For this review, take the finished solid that the model builds, in its own axes (mm). Face numbers are marked on the shaded views. Coordinates: 2 decimals unless noted, no trailing zeros. Write each loop counter-clockwise with the first axis right and the second up, starting at its lowest first coordinate (ties: lowest second). Pieces come first, ordered by that corner, then holes.
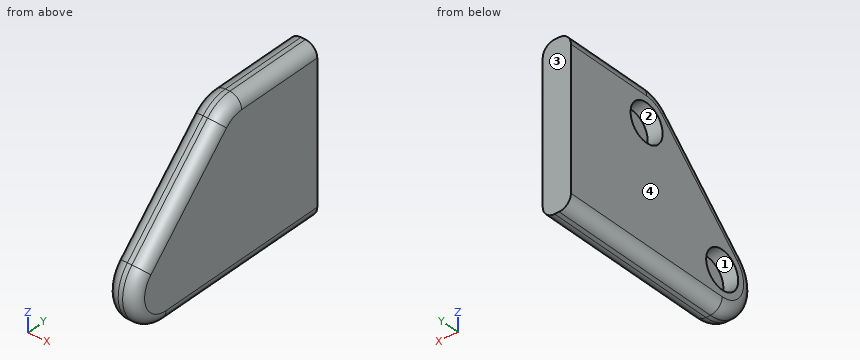
```python
from build123d import *

# Parameters (mm, degrees)
F1_DEPTH = 19
F2_R     = 12.7
F3_DEPTH = 10
F4_R     = 8
F5_R     = 8


with BuildPart() as f1:
    # F0 (on Right) → F1 (new body)
    with BuildSketch(Plane.YZ):
        with BuildLine():
            Line((-120, 0), (0, 0))
            Line((0, 0), (0, 110))
            Line((0, 110), (-60, 110))
            ThreePointArc((-60, 110), (-69.567086, 108.096988), (-77.67767, 102.67767))
            Line((-77.67767, 102.67767), (-137.67767, 42.67767))
            ThreePointArc((-137.67767, 42.67767), (-143.096988, 15.432914), (-120, 0))
        make_face()
    extrude(amount=F1_DEPTH)

    # F2 (on face) → F3 (cut)
    with BuildSketch(Plane(origin=(0, 0, 0), x_dir=(0, -1, 0), z_dir=(-1, 0, 0))):
        with Locations((60, 85)):
            Circle(F2_R)
        with Locations((120, 25)):
            Circle(F2_R)
    extrude(amount=-F3_DEPTH, mode=Mode.SUBTRACT)

    # F4
    f4_edges = [f1.edges().sort_by_distance(p)[0] for p in [
        (0, -30, 110),
    ]]
    fillet(f4_edges, radius=F4_R)

    # F5
    f5_edges = [f1.edges().sort_by_distance(p)[0] for p in [
        (19, -30, 110),
    ]]
    fillet(f5_edges, radius=F5_R)


solid = f1.part
```
Q1. Add section A-A (x = 1.5). State the section outline as (y, z) points, then the cut area to 3 significant figures.
Ans:
outline: (-135.32, 40.32) arc R21.66 ccw to (-120, 3.34) - (0, 3.34) - (0, 106.66) - (-60, 106.66) arc R21.66 ccw to (-75.32, 100.32) - close; hole circle Ø25.4 at (-120, 25); hole circle Ø25.4 at (-60, 85)
area: 10,900 mm2
Q2. Draft analysis for pull direction Y (two halves, no side actions). For the marked faces 1, 2, 3 and 4, state which applies: +Y half, -Y half, draft (parallel to the pull), parting line (faces both ways), or undercut.
Ans:
face 1: undercut
face 2: undercut
face 3: +Y half
face 4: draft
Q3. Add section B-B (y = -40.5). State the section outline as (x, z) points, then the cut area to 3 significant figures.
Ans:
outline: (0, 8) arc R8 ccw to (8, 0) - (11, 0) arc R8 ccw to (19, 8) - (19, 102) arc R8 ccw to (11, 110) - (8, 110) arc R8 ccw to (0, 102) - close
area: 2,040 mm2
Q4. Add section C-C (x = 17.5). State the section outline as (y, z) points.
Ans:
outline: (-135.32, 40.32) arc R21.66 ccw to (-120, 3.34) - (0, 3.34) - (0, 106.66) - (-60, 106.66) arc R21.66 ccw to (-75.32, 100.32) - close
Q5. Clearance check with flat-ended pins moving along their axes: pin 1 Ø6 at (y, z) = (-63, 84.5) entering from -X; pin 2 Ø12 at (y, z) = (-70, 91) entering from -X; pin 3 Ø3 at (x, z) = (6, 70) entering from -Y; pin 4 Ø2 at (y, z) = (-124, 52) entering from +X. State where each tip first meets the part, or that it passes through.
Ans:
pin 1: stops at x = 10
pin 2: stops at x = 0
pin 3: stops at y = -111.57
pin 4: stops at x = 17.97
Q6. For probe 1 along Z at (x, y) = (8.25, -60); probe 2 along Z at (x, y) = (4.5, -60); probe 3 along Y at (x, z) = (6.25, 21), list the stretches that pass through material, from the lowest coordinate up.
Ans:
probe 1: z = 0 to 72.3, 97.7 to 110
probe 2: z = 0.81 to 72.3, 97.7 to 109.19
probe 3: y = -144.48 to -132.05, -107.95 to 0
